Geometry: final body of the model. Coordinates: model frame, mm. Coordinates: 2 decimals unless noted, no trailing zeros. Order: outer loops, then holes, each group sorted by start corner. A loop starts at its lowest first (then second) coordinate and runs counter-clockwise, first axis right, second up. Notation, with made-up numbers: (77, 3) - (102, 3) arc R6 ccw to (102, 8) - close; hole circle Ø4 at (81, 81.5). An arc over 180 degrees is marked (long way). Use a Markdown table: item, result. Add a question column.
```python
from build123d import *

# Parameters (mm, degrees)
BOSS_EXTRUDE2_DEPTH      = 350
BOSS_EXTRUDE2_DEPTH_BACK = 100
SKETCH12_R               = 40
SHELL1_T                 = -10


with BuildPart() as part:
    # Sketch12 → Boss-Extrude2 (new, two sides: drawn at the far end of the back side and taken through both)
    with BuildSketch(Plane(origin=(0, 0, 0), x_dir=(1, 0, 0), z_dir=(0, 1, 0)).offset(-BOSS_EXTRUDE2_DEPTH_BACK)):
        with Locations(Location((0, 0, 0), (0, 0, 270))):
            Circle(SKETCH12_R)
    extrude(amount=BOSS_EXTRUDE2_DEPTH + BOSS_EXTRUDE2_DEPTH_BACK)

    # Shell1
    shell1_openings = [part.faces().sort_by_distance(p)[0] for p in [
        (0, 350, 0),
    ]]
    offset(amount=SHELL1_T, openings=shell1_openings, kind=Kind.INTERSECTION)

    # Cut-Loft1: read off the stored shape, not the designer's step
    # Cut-Loft1: loft between two sections, ruled curve by curve
    cut_loft1_from = [
        Edge.make_bspline([(16.447768561, 299.687176089, 0.756078446), (16.559756866, 299.68551177, 0.757474976), (16.685169468, 299.695855255, 0.748795762), (16.948630904, 299.758019264, 0.696633965), (17.086724057, 299.810484473, 0.652610427), (17.338586824, 299.967314565, 0.521014355), (17.451178642, 300.072155873, 0.433042052), (17.606011876, 300.316064015, 0.22837882), (17.647058824, 300.454214414, 0.112456871), (17.647058824, 300.722256174, -0.112456871), (17.606011876, 300.860406573, -0.22837882), (17.451178642, 301.104314716, -0.433042052), (17.338586824, 301.209156023, -0.521014355), (17.086724057, 301.365986115, -0.652610427), (16.948630904, 301.418451325, -0.696633965), (16.685169468, 301.480615333, -0.748795762), (16.559756866, 301.490958819, -0.757474976), (16.447768561, 301.489294499, -0.756078446)], [0, 0, 0, 0, 0.125, 0.125, 0.25, 0.25, 0.375, 0.375, 0.5, 0.5, 0.625, 0.625, 0.75, 0.75, 0.875, 0.875, 1, 1, 1, 1], 3),
        Edge.make_bspline([(16.447768561, 301.489294499, -0.756078446), (14.881581053, 332.389152096, -26.684137559), (-14.881581053, 332.389152096, -26.684137559), (-16.447768561, 301.489294499, -0.756078446)], [0, 0, 0, 0, 1, 1, 1, 1], 3, [1, 0.368414451, 0.368414451, 1]),
        Edge.make_bspline([(-16.447768561, 299.687176089, 0.756078446), (-14.881581053, 268.787318493, 26.684137559), (14.881581053, 268.787318493, 26.684137559), (16.447768561, 299.687176089, 0.756078446)], [0, 0, 0, 0, 1, 1, 1, 1], 3, [1, 0.368414451, 0.368414451, 1]),
        Edge.make_bspline([(-16.447768561, 301.489294499, -0.756078446), (-16.559756866, 301.490958819, -0.757474976), (-16.685169468, 301.480615333, -0.748795762), (-16.948630904, 301.418451325, -0.696633965), (-17.086724057, 301.365986115, -0.652610427), (-17.338586824, 301.209156023, -0.521014355), (-17.451178642, 301.104314716, -0.433042052), (-17.606011876, 300.860406573, -0.22837882), (-17.647058824, 300.722256174, -0.112456871), (-17.647058824, 300.454214414, 0.112456871), (-17.606011876, 300.316064015, 0.22837882), (-17.451178642, 300.072155873, 0.433042052), (-17.338586824, 299.967314565, 0.521014355), (-17.086724057, 299.810484473, 0.652610427), (-16.948630904, 299.758019264, 0.696633965), (-16.685169468, 299.695855255, 0.748795762), (-16.559756866, 299.68551177, 0.757474976), (-16.447768561, 299.687176089, 0.756078446)], [0, 0, 0, 0, 0.125, 0.125, 0.25, 0.25, 0.375, 0.375, 0.5, 0.5, 0.625, 0.625, 0.75, 0.75, 0.875, 0.875, 1, 1, 1, 1], 3),
    ]
    cut_loft1_to = [
        Edge.make_bspline([(17.602105154, 396.042079443, 115.71580798), (17.609587889, 396.12223285, 115.648551286), (17.616135283, 396.20246302, 115.58123018), (17.627359386, 396.363038504, 115.44649135), (17.632036096, 396.443383819, 115.379073626), (17.639518831, 396.604151212, 115.244173766), (17.642324857, 396.68457329, 115.17669163), (17.646066225, 396.845455828, 115.041695152), (17.647001567, 396.925916287, 114.97418081), (17.647001567, 397.086837207, 114.839152126), (17.646066225, 397.167297667, 114.771637784), (17.642324857, 397.328180204, 114.636641306), (17.639518831, 397.408602282, 114.569159169), (17.632036096, 397.569369675, 114.434259309), (17.627359386, 397.64971499, 114.366841585), (17.616135283, 397.810290475, 114.232102756), (17.609587889, 397.890520644, 114.16478165), (17.602105154, 397.970674051, 114.097524956)], [0, 0, 0, 0, 0.125, 0.125, 0.25, 0.25, 0.375, 0.375, 0.5, 0.5, 0.625, 0.625, 0.75, 0.75, 0.875, 0.875, 1, 1, 1, 1], 3),
        Edge.make_bspline([(17.602105154, 397.970674051, 114.097524956), (15.404444247, 421.511531348, 94.34440028), (-15.404444247, 421.511531348, 94.34440028), (-17.602105154, 397.970674051, 114.097524956)], [0, 0, 0, 0, 1, 1, 1, 1], 3, [1, 0.380888028, 0.380888028, 1]),
        Edge.make_bspline([(-17.602105154, 396.042079443, 115.71580798), (-15.404444247, 372.501222146, 135.468932655), (15.404444247, 372.501222146, 135.468932655), (17.602105154, 396.042079443, 115.71580798)], [0, 0, 0, 0, 1, 1, 1, 1], 3, [1, 0.380888028, 0.380888028, 1]),
        Edge.make_bspline([(-17.602105154, 397.970674051, 114.097524956), (-17.609587889, 397.890520644, 114.16478165), (-17.616135283, 397.810290475, 114.232102756), (-17.627359386, 397.64971499, 114.366841585), (-17.632036096, 397.569369675, 114.434259309), (-17.639518831, 397.408602282, 114.569159169), (-17.642324857, 397.328180204, 114.636641306), (-17.646066225, 397.167297667, 114.771637784), (-17.647001567, 397.086837207, 114.839152126), (-17.647001567, 396.925916287, 114.97418081), (-17.646066225, 396.845455828, 115.041695152), (-17.642324857, 396.68457329, 115.17669163), (-17.639518831, 396.604151212, 115.244173766), (-17.632036096, 396.443383819, 115.379073626), (-17.627359386, 396.363038504, 115.44649135), (-17.616135283, 396.20246302, 115.58123018), (-17.609587889, 396.12223285, 115.648551286), (-17.602105154, 396.042079443, 115.71580798)], [0, 0, 0, 0, 0.125, 0.125, 0.25, 0.25, 0.375, 0.375, 0.5, 0.5, 0.625, 0.625, 0.75, 0.75, 0.875, 0.875, 1, 1, 1, 1], 3),
    ]
    cut_loft1 = Solid(Shell([*[Face.make_surface_from_curves(cut_loft1_from[k], cut_loft1_to[k]) for k in range(4)], Face(Wire(cut_loft1_from)), Face(Wire(cut_loft1_to))]))
    add(cut_loft1, mode=Mode.SUBTRACT)

    # Sketch15 → Cut-Loft3 section 0
    with BuildSketch(Plane.XY):
        with BuildLine():
            Line((-16.470588235, 350), (16.470588235, 350))
            Line((16.470588235, 350), (16.470588235, 300.588235294))
            Line((16.470588235, 300.588235294), (-16.470588235, 300.588235294))
            Line((-16.470588235, 300.588235294), (-16.470588235, 350))
        make_face()
    # Sketch20 → Cut-Loft3 section 1
    with BuildSketch(Plane(origin=(0, 397.006376747, 114.906666468), x_dir=(1, 0, 0), z_dir=(0, 0.6427876096865435, 0.7660444431189747))):
        with BuildLine():
            Line((-17.647058824, 0), (-17.647058824, 17.647058824))
            Line((-17.647058824, 17.647058824), (17.647058824, 17.647058824))
            Line((17.647058824, 17.647058824), (17.647058824, 0))
            ThreePointArc((17.647058824, 0), (0, -17.647058824), (-17.647058824, 0))
        make_face()
    loft(mode=Mode.SUBTRACT)


solid = part.part
```
1) Section A-A (z = 0). Return loops of the section in (x, y), then the cut area to 3 significant figures.
2) Ray query, line 1 along Z through (x, y) = (0, 123); line 2 along Y through (x, z) = (6, 28.5). Return the intervals inside material, ascending.
3) Section B-B (y = -38.5). Return loops of the section in (x, z).
4) Draft query along Z for faces 1 (the face through (1, -100, -1)), 2 (the face through (1.32, 126.92, -29.97)), 3 (the face through (0, -90, 0)), 4 (the face through (1.76, 121.85, -39.96)). Return one class per face: pulls with the +Z half, pulls with the -Z half, needs draft (parallel to the pull), parting line crosses it, or undercut.
5) Pin query (flat end, axial travel): pin 1 (1.5 mm diameter, centred on x = 26, y = 106.5, fed in from +Z); pin 2 (1 mm diameter, centred on y = 213, z = 21, fed in from +X); pin 3 (12 mm diameter, centred on x = 13.5, z = 0, fed in from +Y). Return the tip coordinate at first contact, or that it passes through.
Values follow:
| question | item | result |
|---|---|---|
| 1 | outline | (-40, -100) - (40, -100) - (40, 350) - (30, 350) - (30, -90) - (-30, -90) - (-30, 350) - (-40, 350) - close |
| 1 | area | 9,600 mm² |
| 2 | line 1 | z = -40 to -30, 30 to 40 |
| 2 | line 2 | y = -100 to -90 |
| 3 | outline | circle Ø80 at (0, 0); hole circle Ø60 at (0, 0) |
| 4 | face 1 | needs draft |
| 4 | face 2 | undercut |
| 4 | face 3 | undercut |
| 4 | face 4 | parting line crosses it |
| 5 | pin 1 | stops at z = 31.02 |
| 5 | pin 2 | stops at x = 34.35 |
| 5 | pin 3 | stops at y = -90 |
